Geometry check sheet. Reference: the model listing, model coordinates, mm. Face numbers are marked on the shaded views. A direction names the side the tool comes from. Coordinates: 2 decimals unless noted, no trailing zeros. Write each loop counter-clockwise with the first axis right and the second up, starting at its lowest first coordinate (ties: lowest second). Pieces come first, ordered by that corner, then holes. Notation, with made-up numbers: (74, 65.5) -> (118, 65.5) arc R16 cw to (118, 88.5) -> close; hole circle Ø7 at (-32, 45). An arc over 180 degrees is marked (long way). Answer in a Markdown table with one row per item. Add a question column.
1. Mould release check, pull along X, two halves, no side actions. Record for the marked faces 5, 6 and 7: pulls with the +X half, pulls with the -X half, needs draft (parallel to the pull), parting line crosses it, or undercut.
2. Cross-section at C-C on y = 39. Record the cut outline in (x, z).
3. Cross-section at A-A on z = 13. Give the number of separate pieces and of enclosed holes in the cut face, and give its area (3 significant figures).
4. Set-up check for the marked faces 1, 2, 3 and 4: record each of +Z, -Z, +X, -X, +Y, -Y from which the full face is reachable in a straight line by a thin tool's end or side.
5. Depth check by flat-ended pin: P1, Ø5, axis at y = 24, z = 15, coming from the -X side; P2, Ø7.5, axis at y = -10, z = 16.5, coming from the -X side; P3, Ø5, axis at y = 53.5, z = 15.5, coming from the +X side. Enter the tip coordinate at first touch or a pass-through.
6. Cross-section at B-B on y = 60. Record the cut outline in (x, z), and give its area (3 significant figures).
7. Scan lines: L1, parallel to Z at x = -1, y = 60; L2, parallel to X at y = -6, z = 23; L3, parallel to X at y = 43.5, z = 17. Record each from-to range of solid material in increasing order. Write a range as from..to.
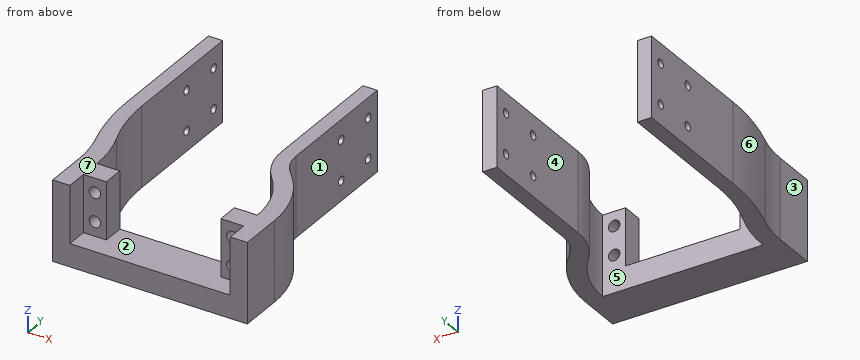
```python
from build123d import *

# Parameters (mm, degrees)
SKETCH1_W           = 8
SKETCH1_H           = 8
SKETCH1_W_2         = 40
BOSS_EXTRUDE1_DEPTH = 15
SKETCH1_5_W         = 8
SKETCH1_5_H         = 20
SKETCH1_5_R         = 2
BOSS_EXTRUDE2_DEPTH = 7.5
BOSS_EXTRUDE3_DEPTH = 28
CUT_EXTRUDE1_REACH  = 105.271
SKETCH3_R           = 1.5


with BuildPart() as part:
    # Sketch1 → Boss-Extrude1 (new body)
    with BuildSketch(Plane(origin=(0, 0, 0), x_dir=(1, 0, 0), z_dir=(0, 1, 0))):
        Polygon((6, -28), (6, -8), (6, 0), (0, 0), (0, -28), align=None)
        with Locations((10, -4)):
            Rectangle(SKETCH1_W, SKETCH1_H)
        with Locations((34, -4)):
            Rectangle(SKETCH1_W_2, SKETCH1_H)
        with Locations((58, -4)):
            Rectangle(SKETCH1_W, SKETCH1_H)
        Polygon((62, 0), (62, -8), (62, -28), (68, -28), (68, 0), align=None)
    extrude(amount=-BOSS_EXTRUDE1_DEPTH)

    # Sketch1<5> → Boss-Extrude2 (add)
    # profile 1 of 2: a face of its own
    with BuildSketch(Plane(origin=(0, 0, 0), x_dir=(1, 0, 0), z_dir=(0, 1, 0))):
        with Locations((10, -18)):
            Rectangle(SKETCH1_5_W, SKETCH1_5_H)
        with Locations(Location((10, -23, 0), (0, 0, 270))):
            Circle(SKETCH1_5_R, mode=Mode.SUBTRACT)
        with Locations(Location((10, -13, 0), (0, 0, 270))):
            Circle(SKETCH1_5_R, mode=Mode.SUBTRACT)
    # profile 2 of 2: a face of its own
    with BuildSketch(Plane(origin=(0, 0, 0), x_dir=(1, 0, 0), z_dir=(0, 1, 0))):
        with Locations((58, -18)):
            Rectangle(SKETCH1_5_W, SKETCH1_5_H)
        with Locations(Location((58, -23, 0), (0, 0, 270))):
            Circle(SKETCH1_5_R, mode=Mode.SUBTRACT)
        with Locations(Location((58, -13, 0), (0, 0, 270))):
            Circle(SKETCH1_5_R, mode=Mode.SUBTRACT)
    extrude(amount=-BOSS_EXTRUDE2_DEPTH)

    # Sketch2 → Boss-Extrude3 (add)
    with BuildSketch(Plane.XY.offset(28)):
        with BuildLine():
            Line((-0.5, 80), (-5.5, 80))
            Line((-5.5, 80), (-5.5, 35))
            ThreePointArc((-5.5, 35), (-4.567837418, 23.063317904), (-1.793950653, 11.416049609))
            ThreePointArc((-1.793950653, 11.416049609), (-0.451222721, 5.778071643), (0, 0))
            Line((0, 0), (6, 0))
            ThreePointArc((6, 0), (5.273404236, 7.891775129), (3.118046932, 15.51820883))
            ThreePointArc((3.118046932, 15.51820883), (0.412179175, 25.092547618), (-0.5, 35))
            Line((-0.5, 35), (-0.5, 80))
        make_face()
        with BuildLine():
            Line((53.5, 80), (48.5, 80))
            Line((48.5, 80), (48.5, 35))
            ThreePointArc((48.5, 35), (49.937115956, 27.280735927), (54.055895054, 20.595827638))
            ThreePointArc((54.055895054, 20.595827638), (59.945137576, 11.037401409), (62, 0))
            Line((62, 0), (68, 0))
            ThreePointArc((68, 0), (65.207771721, 14.035220845), (57.256309947, 25.933044956))
            ThreePointArc((57.256309947, 25.933044956), (54.476245108, 30.092874105), (53.5, 35))
            Line((53.5, 35), (53.5, 80))
        make_face()
    extrude(amount=-BOSS_EXTRUDE3_DEPTH)

    # Cut-Extrude1: up to this face of the body (flat: up to its plane)
    cut_extrude1_end = Plane(part.part.faces().sort_by_distance((-5.5, 57.5, 14))[0])
    # Sketch3 → Cut-Extrude1 (cut, up to the picked face)
    with BuildSketch(Plane(origin=(53.5, 0, 0), x_dir=(0, 0, -1), z_dir=(1, 0, 0)), mode=Mode.PRIVATE) as cut_extrude1_sk1:
        with Locations(Location((-21, 75, 0), (0, 0, 90))):
            Circle(SKETCH3_R)
    cut_extrude1_tool1 = split(extrude(cut_extrude1_sk1.sketch, amount=-CUT_EXTRUDE1_REACH, mode=Mode.PRIVATE), bisect_by=cut_extrude1_end, keep=Keep.BOTH, mode=Mode.PRIVATE)
    # Sketch3 → Cut-Extrude1 (cut, up to the picked face)
    with BuildSketch(Plane(origin=(53.5, 0, 0), x_dir=(0, 0, -1), z_dir=(1, 0, 0)), mode=Mode.PRIVATE) as cut_extrude1_sk2:
        with Locations(Location((-21, 60, 0), (0, 0, 90))):
            Circle(SKETCH3_R)
    cut_extrude1_tool2 = split(extrude(cut_extrude1_sk2.sketch, amount=-CUT_EXTRUDE1_REACH, mode=Mode.PRIVATE), bisect_by=cut_extrude1_end, keep=Keep.BOTH, mode=Mode.PRIVATE)
    # Sketch3 → Cut-Extrude1 (cut, up to the picked face)
    with BuildSketch(Plane(origin=(53.5, 0, 0), x_dir=(0, 0, -1), z_dir=(1, 0, 0)), mode=Mode.PRIVATE) as cut_extrude1_sk3:
        with Locations(Location((-7, 60, 0), (0, 0, 180))):
            Circle(SKETCH3_R)
    cut_extrude1_tool3 = split(extrude(cut_extrude1_sk3.sketch, amount=-CUT_EXTRUDE1_REACH, mode=Mode.PRIVATE), bisect_by=cut_extrude1_end, keep=Keep.BOTH, mode=Mode.PRIVATE)
    # Sketch3 → Cut-Extrude1 (cut, up to the picked face)
    with BuildSketch(Plane(origin=(53.5, 0, 0), x_dir=(0, 0, -1), z_dir=(1, 0, 0)), mode=Mode.PRIVATE) as cut_extrude1_sk4:
        with Locations(Location((-7, 75, 0), (0, 0, 180))):
            Circle(SKETCH3_R)
    cut_extrude1_tool4 = split(extrude(cut_extrude1_sk4.sketch, amount=-CUT_EXTRUDE1_REACH, mode=Mode.PRIVATE), bisect_by=cut_extrude1_end, keep=Keep.BOTH, mode=Mode.PRIVATE)
    add(cut_extrude1_tool1.solids().sort_by(Axis((53.5, 75, 21), (-1, 0, 0)))[0], mode=Mode.SUBTRACT)
    add(cut_extrude1_tool2.solids().sort_by(Axis((53.5, 60, 21), (-1, 0, 0)))[0], mode=Mode.SUBTRACT)
    add(cut_extrude1_tool3.solids().sort_by(Axis((53.5, 60, 7), (-1, 0, 0)))[0], mode=Mode.SUBTRACT)
    add(cut_extrude1_tool4.solids().sort_by(Axis((53.5, 75, 7), (-1, 0, 0)))[0], mode=Mode.SUBTRACT)


solid = part.part
```
Results found:
| question | item | result |
|---|---|---|
| 1 | face 5 | undercut |
| 1 | face 6 | pulls with the -X half |
| 1 | face 7 | needs draft |
| 2 | outline | (-5.5, 0) -> (-0.5, 0) -> (-0.5, 28) -> (-5.5, 28) -> close; (48.5, 0) -> (53.5, 0) -> (53.5, 28) -> (48.5, 28) -> close |
| 3 | separate pieces | 4 |
| 3 | enclosed holes | 0 |
| 3 | area | 1,110 mm^2 |
| 4 | face 1 | +Z, -Z, +X, +Y |
| 4 | face 2 | +Z, -Y |
| 4 | face 3 | +Z, -Z, -X, -Y |
| 4 | face 4 | +Z, -Z, +Y |
| 5 | P1 | stops at x = -5.03 |
| 5 | P2 | stops at x = 0 |
| 5 | P3 | stops at x = 53.5 |
| 6 | outline | (-5.5, 0) -> (-0.5, 0) -> (-0.5, 5.5) -> (-5.5, 5.5) -> close; (-5.5, 8.5) -> (-0.5, 8.5) -> (-0.5, 19.5) -> (-5.5, 19.5) -> close; (-5.5, 22.5) -> (-0.5, 22.5) -> (-0.5, 28) -> (-5.5, 28) -> close; (48.5, 0) -> (53.5, 0) -> (53.5, 5.5) -> (48.5, 5.5) -> close; (48.5, 8.5) -> (53.5, 8.5) -> (53.5, 19.5) -> (48.5, 19.5) -> close; (48.5, 22.5) -> (53.5, 22.5) -> (53.5, 28) -> (48.5, 28) -> close |
| 6 | area | 220 mm^2 |
| 7 | L1 | z = 0..5.5, 8.5..19.5, 22.5..28 |
| 7 | L2 | x = 0..8, 12..14, 54..56, 60..68 |
| 7 | L3 | x = -5.5..-0.5, 48.5..53.5 |
